from build123d import *

# Parameters (mm, degrees)
F0_R     = 3.81
F1_DEPTH = 5.08
F2_R     = 3.175
F3_R     = 1.27
F4_DEPTH = 3.81
F5_R     = 1.909408
F6_DEPTH = 1.27


with BuildPart() as f1:
    # F0 (on Top) → F1 (new body)
    with BuildSketch(Plane.XY):
        Circle(F0_R)
    extrude(amount=F1_DEPTH)

    # F2
    f2_edges = [f1.edges().sort_by_distance(p)[0] for p in [
        (-3.81, 0, 0),
    ]]
    fillet(f2_edges, radius=F2_R)

    # F3 (on face) → F4 (join)
    with BuildSketch(Plane.XY.offset(5.08)):
        Circle(F3_R)
    extrude(amount=F4_DEPTH)

    # F5 (on face) → F6 (join)
    with BuildSketch(Plane.XY.offset(5.08)):
        Circle(F5_R)
    extrude(amount=F6_DEPTH)


solid = f1.part
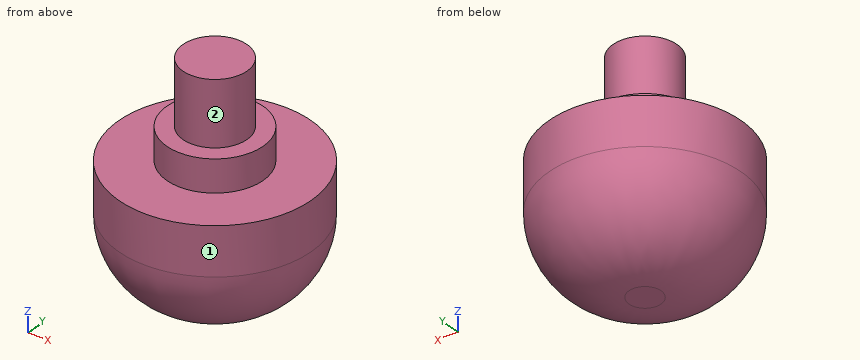
Read the model definition and answer for the solid it produces. Units are mm, in the model's axes. Face numbers are marked on the shaded views. A direction names the side the tool comes from. Round coordinates to 2 decimals unless told otherwise and drop trailing zeros. Write each loop counter-clockwise with the first axis right and the second up, starting at its lowest first coordinate (ties: lowest second). Pieces come first, ordered by that corner, then holes.
Q1. Find section B-B on z = 7.75. Determine the outline of the cut face in (x, y).
Values:
outline: circle Ø2.54 at (0, 0)
Q2. Flat-ended cylindrical pins translate along their axes: P1, Ø1.5, axis at y = -2, z = 3.5, coming from the -X side; P2, Ø1.5, axis at x = -2, z = 2, coming from the +Y side; P3, Ø2, axis at x = -2, z = 2, coming from the -Y side; P4, Ø4, axis at x = -1, y = 1.5, coming from the +Z side. Find the tip coordinate at first contact, or state that the pin passes through.
Values:
P1: stops at x = -3.6
P2: stops at y = 3.45
P3: stops at y = -3.56
P4: stops at z = 8.89
Q3. A tool of negligible diameter and unlimited length cuts with its end or side. For the marked faces 1 and 2, from which of +Z, -Z, +X, -X, +Y, -Y can it reach the whole face along a straight path? Write none if from no direction.
Values:
face 1: +Z, -Z
face 2: +Z
Q4. Straight lines are drawn through the part: line 1 (Y direction, x = 0.25, z = 6.75); line 2 (Y direction, x = 3, z = 4.25); line 3 (Z direction, x = 3, y = -1.25). For each, find the intervals that lie inside material, in ascending order.
Values:
line 1: y = -1.25 to 1.25
line 2: y = -2.35 to 2.35
line 3: z = 1.37 to 5.08
Q5. Find section A-A on z = 3.75. Determine the outline of the cut face in (x, y), and give its area (3 significant figures).
Values:
outline: circle Ø7.62 at (0, 0)
area: 45.6 mm2
